```python
from build123d import *

# Parameters (mm, degrees)
SKETCH1_W           = 20
SKETCH1_H           = 48
BOSS_EXTRUDE1_DEPTH = 5
SKETCH2_R           = 3.5
CUT_EXTRUDE1_DEPTH  = 27.47640459
SKETCH3_R           = 5
CUT_EXTRUDE2_DEPTH  = 3
SKETCH4_R           = 1.5
CUT_EXTRUDE3_DEPTH  = 27.47640459


with BuildPart() as part:
    # Sketch1 → Boss-Extrude1 (new body)
    with BuildSketch(Plane(origin=(0, 0, 0), x_dir=(1, 0, 0), z_dir=(0, 1, 0))):
        Rectangle(SKETCH1_W, SKETCH1_H)
    extrude(amount=BOSS_EXTRUDE1_DEPTH)

    # Sketch2 → Cut-Extrude1 (cut, through all)
    with BuildSketch(Plane(origin=(0, 5, 0), x_dir=(1, 0, 0), z_dir=(0, 1, 0))):
        with Locations(Location((0, 0, 0), (0, 0, 270))):
            Circle(SKETCH2_R)
    extrude(amount=-CUT_EXTRUDE1_DEPTH, mode=Mode.SUBTRACT)

    # Sketch3 → Cut-Extrude2 (cut)
    with BuildSketch(Plane.XZ):
        with Locations(Location((0, 0, 0), (0, 0, 270))):
            Circle(SKETCH3_R)
    extrude(amount=-CUT_EXTRUDE2_DEPTH, mode=Mode.SUBTRACT)

    # Sketch4 → Cut-Extrude3 (cut, through all)
    with BuildSketch(Plane.XZ):
        with Locations(Location((5, -16.5, 0), (0, 0, 270))):
            Circle(SKETCH4_R)
        with Locations(Location((-5, -16.5, 0), (0, 0, 270))):
            Circle(SKETCH4_R)
        with Locations(Location((-5, 16.5, 0), (0, 0, 270))):
            Circle(SKETCH4_R)
        with Locations(Location((5, 16.5, 0), (0, 0, 270))):
            Circle(SKETCH4_R)
    extrude(amount=-CUT_EXTRUDE3_DEPTH, mode=Mode.SUBTRACT)


solid = part.part
```
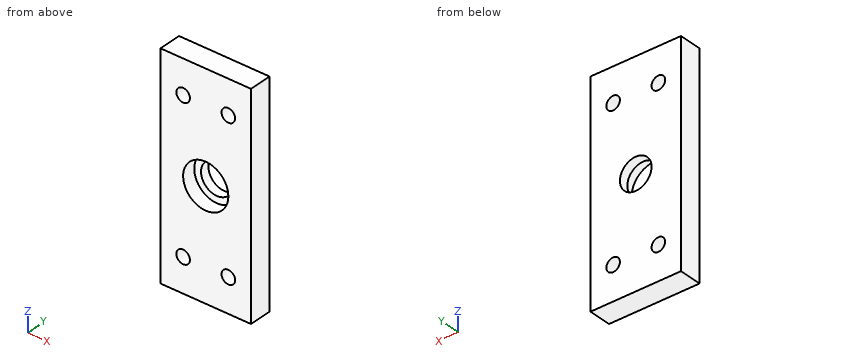
Work out the finished part from the listing and answer in its coordinate system (mm). Coordinates: 2 decimals unless noted, no trailing zeros. Order: outer loops, then holes, each group sorted by start corner. A loop starts at its lowest first (then second) coordinate and runs counter-clockwise, first axis right, second up. Notation, with made-up numbers: M 0,15 L 32,15 A15 ccw 32,20 Z; hole C 12,-30.5 d8. An arc over 180 degrees is marked long. Use CSV: the item, a comma, the result in double quotes.
1) Consider line 1 (X direction, y = 3.15, z = 16.5); line 2 (X direction, y = 1.5, z = -17.5); line 3 (X direction, y = 4.45, z = 0). Determine where each line is inside the solid, lowest interval first. Write a range as [from, to].
Worked out:
line 1,"x = [-10, -6.5], [-3.5, 3.5], [6.5, 10]"
line 2,"x = [-10, -6.12], [-3.88, 3.88], [6.12, 10]"
line 3,"x = [-10, -3.5], [3.5, 10]"
2) Section A-A on z = 0 is taken. Write down the section's boundary in (x, y).
Worked out:
outline,"M -10,0 L -5,0 L -5,3 L -3.5,3 L -3.5,5 L -10,5 Z; M 3.5,3 L 5,3 L 5,0 L 10,0 L 10,5 L 3.5,5 Z"
3) Section D-D on x = 3 is taken. Write down the section's boundary in (y, z).
Worked out:
outline,"M 0,-24 L 5,-24 L 5,-1.8 L 3,-1.8 L 3,-4 L 0,-4 Z; M 0,4 L 3,4 L 3,1.8 L 5,1.8 L 5,24 L 0,24 Z"
4) Section C-C on y = 4.15 is taken. Write down the section's boundary in (x, z).
Worked out:
outline,"M -10,-24 L 10,-24 L 10,24 L -10,24 Z; hole C -5,-16.5 d3; hole C -5,16.5 d3; hole C 0,0 d7; hole C 5,-16.5 d3; hole C 5,16.5 d3"
5) Section B-B on z = 16.5 is taken. Write down the section's boundary in (x, y), plus the area to 3 significant figures.
Worked out:
outline,"M -10,0 L -6.5,0 L -6.5,5 L -10,5 Z; M -3.5,0 L 3.5,0 L 3.5,5 L -3.5,5 Z; M 6.5,0 L 10,0 L 10,5 L 6.5,5 Z"
area,"70.0 mm^2"
6) A flat-ended cylindrical pin translates along its axis: pin 1 Ø4 at (x, z) = (0, 0) entering from +Y. Find the tip coordinate at first contact, or state that the pin passes through.
Worked out:
pin 1,"passes through"
